Geometry: see drawing. Coordinates: mm, zero at the bounding-box minimum. A direction names the side the tool comes from. Coordinates: 2 decimals unless noted, no trailing zeros. Write each loop counter-clockwise with the first axis right and the second up, starting at its lowest first coordinate (ties: lowest second). Pieces come first, ordered by that corner, then holes. Notation, with made-up numbers: M -3.5,38.5 L 42.5,38.5 A26 cw 42.5,67.5 Z; hole C 73,32 d1. An arc over 180 degrees is marked long. Write item = value, one per line. Start each with the question number.
1. Section query A-A (y = 10). Output: boundary loops of the cut face in (x, z), then the cut area to 4 significant figures.
2. Section query C-C (x = 10). Output: boundary loops of the cut face in (y, z), then the cut area to 3 significant figures.
3. Access query for the marked faces 4 and 5. Directions: +Z, -Z, +X, -X, +Y, -Y. A direction counts if a zero-diameter tool reaches every point of the face in a straight line with its end or side. Return the directions, or none.
4. Line query: line 1 along X through (y, z) = (9, 4.75); line 2 along Z through (x, y) = (14.5, 5); line 3 along Y through (x, z) = (10, 0.8). Output: solid intervals per line, ascending.
5. Pull-direction query (Z, two-part tool) for the marked faces 1, 2 and 3; classes: pulls with the +Z half, pulls with the -Z half, needs draft (parallel to the pull), parting line crosses it, or undercut.
6. Section query D-D (z = 13.75). Output: boundary loops of the cut face in (x, y).
7. Pin query (flat end, axial travel): pin 1 Ø12 at (x, y) = (9.5, 15.5) entering from +Z; pin 2 Ø5 at (x, y) = (3.5, 15.5) entering from +Z; pin 3 Ø4.5 at (x, z) = (10, 10) entering from +Y; pin 4 Ø3 at (x, y) = (10, 10) entering from +Z. Return the tip coordinate at first contact, or that it passes through.
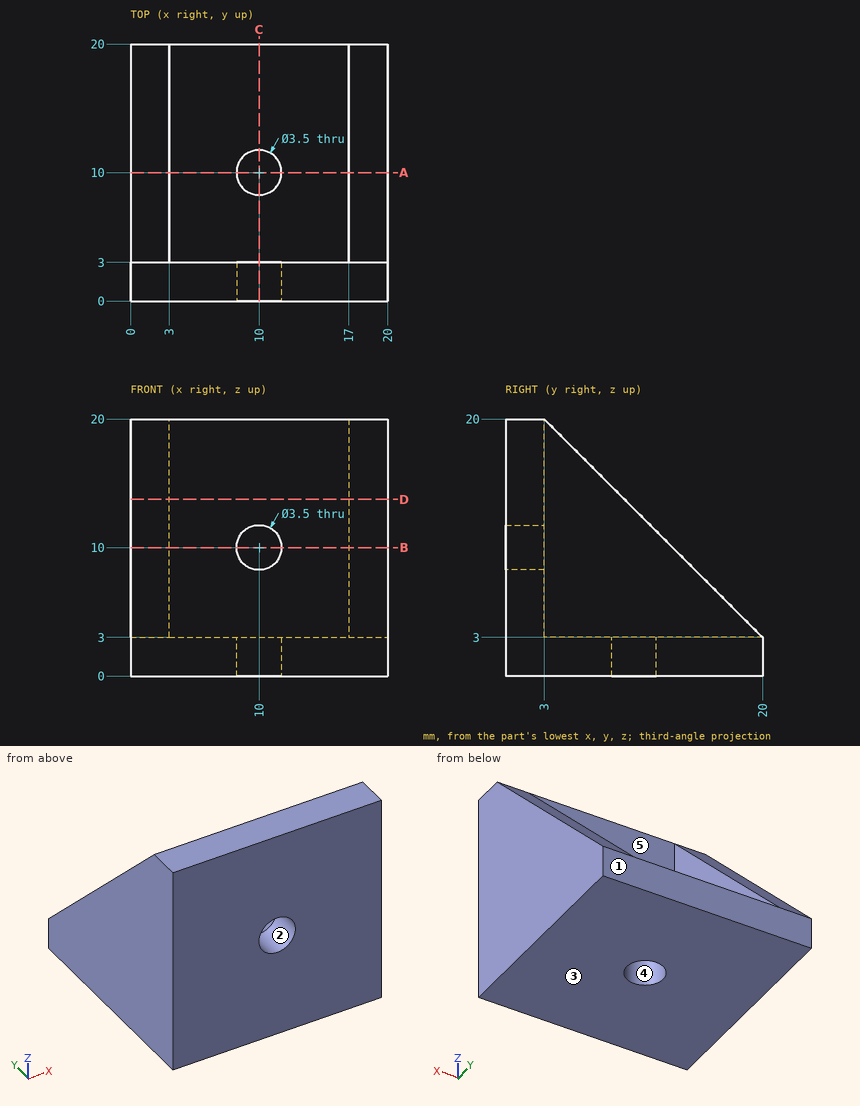
Results are:
q1.outline = M 0,0 L 8.25,0 L 8.25,3 L 3,3 L 3,13 L 0,13 Z; M 11.75,0 L 20,0 L 20,13 L 17,13 L 17,3 L 11.75,3 Z
q1.area = 109.5 mm^2
q2.outline = M 0,0 L 8.25,0 L 8.25,3 L 3,3 L 3,8.25 L 0,8.25 Z; M 0,11.75 L 3,11.75 L 3,20 L 0,20 Z; M 11.75,0 L 20,0 L 20,3 L 11.75,3 Z
q2.area = 90.0 mm^2
q3.face_4 = +Z, -Z
q3.face_5 = +Z, +Y
q4.line_1 = 0 to 3, 17 to 20
q4.line_2 = 0 to 3
q4.line_3 = 0 to 8.25, 11.75 to 20
q5.face_1 = needs draft
q5.face_2 = undercut
q5.face_3 = pulls with the -Z half
q6.outline = M 0,0 L 20,0 L 20,9.25 L 17,9.25 L 17,3 L 3,3 L 3,9.25 L 0,9.25 Z
q7.pin_1 = 3
q7.pin_2 = 9.95
q7.pin_3 = 3
q7.pin_4 = through
